For this review, take the finished solid that the model builds, in its own axes (mm). A direction names the side the tool comes from. Round coordinates to 2 decimals unless told otherwise and drop trailing zeros. Loops run counter-clockwise (first coordinate to the right, second up) from the corner with the lowest first, then second, coordinate; pieces in that order, holes last. Notation, with made-up numbers: M 70,-13.75 L 123,-13.75 A26 cw 123,6.25 Z; hole C 47,73 d8. An arc over 180 degrees is marked long. Write item = value, one per line. Start each with the question number.
Autodesk Inventor part; units mm, degrees
ref_plane "YZ Plane" through (0, 0, 0) normal (1, 0, 0) x (0, 1, 0)
ref_plane "XZ Plane" through (0, 0, 0) normal (0, 1, 0) x (-1, 0, 0)
ref_plane "XY Plane" through (0, 0, 0) normal (0, 0, 1) x (1, 0, 0)
sketch "Эскиз1" plane through (0, 0, 0) normal (0, 0, 1) x (1, 0, 0)
  line L0 (80, 0) -> (-80, 0) construction
  line L1 (80, 15) -> (-80, 15)
  line L2 (-80, -15) -> (80, -15)
  arc A0 (80, -15) -> (80, 15) centre (80, 0) ccw
  arc A1 (-80, 15) -> (-80, -15) centre (-80, 0) ccw
  circle A2 centre (0, 0) radius 12.5
  circle A3 centre (0, 0) radius 6
  circle A4 centre (-80, 0) radius 5
  circle A5 centre (80, 0) radius 5
  dimension "d0" = 80
  dimension "d1" = 30
  dimension "d4" = 25
  dimension "d5" = 12
  dimension "d6" = 10
  dimension "d7" = 10
extrude "Выдавливание1" add sketch "Эскиз1" against normal blind 10 contours A0 L2 A1 L1 | A2 | A3 | A4 | A5
extrude "Выдавливание2" cut sketch "Эскиз1" against normal blind 10 contours A5
extrude "Выдавливание3" cut sketch "Эскиз1" against normal blind 10 contours A4
extrude "Выдавливание4" add sketch "Эскиз1" along normal blind 20 contours A2
extrude "Выдавливание5" cut sketch "Эскиз1" along normal mid plane 2850 contours A3
equation "\"Глубина_просечки\" = 0.5 * Толщина"
properties part number "крышка" material "Сталь"
(1) Add section C-C on x = 0. Write out the cut boundary in (y, z).
(2) Add section B-B on y = 0. Write out the cut boundary in (x, z), and give its area (3 significant figures).
(3) Add section A-A on z = -3.25. Write out the cut boundary in (x, y).
(4) Wall thickness on L1, parallel to Y at x = -80, z = -6.5; L2, parallel to Z at x = -38.5, y = 8.75; L3, parallel to X at y = -2, z = 9.25: over which ranges is each line inside the solid? List them lowest first.
(5) For pin 1 Ø3 at (y, z) = (11, 3.5) entering from -X; pin 2 Ø10 at (x, y) = (53.5, -5.5) entering from +Z; pin 3 Ø1 at (y, z) = (-7, -2.5) entering from +X, all flat-tipped, find the tip position at first contact; note any pin that passes through.
(6) Add section D-D on z = 4.75. Write out the cut boundary in (x, y), and give its area (3 significant figures).
(7) Tool access review of faces 5 (the cylindrical face through (11.923, -3.755, 9.86)), 6 (the flat face through (1, 15, -5)): name each direction out of +Z, -Z, +X, -X, +Y, -Y from which nothing blocks a thin tool from reaching the whole face with its end or side.
(8) Draft analysis for pull direction Y (two halves, no side actions). For faces 1 (the cylindrical face through (84.619, -1.915, -4.93)), 2 (the flat face through (-1, -15, -5)), 3 (the flat face through (-3, -5.4, 20)), 4 (the cylindrical face through (-95, 0, -5)), state which applies: +Y half, -Y half, draft (parallel to the pull), parting line (faces both ways), or undercut.
Answer sheet:
q1.outline = M -15,-10 L -6,-10 L -6,20 L -12.5,20 L -12.5,0 L -15,0 Z; M 6,-10 L 15,-10 L 15,0 L 12.5,0 L 12.5,20 L 6,20 Z
q2.outline = M -95,-10 L -85,-10 L -85,0 L -95,0 Z; M -75,-10 L -6,-10 L -6,20 L -12.5,20 L -12.5,0 L -75,0 Z; M 6,-10 L 75,-10 L 75,0 L 12.5,0 L 12.5,20 L 6,20 Z; M 85,-10 L 95,-10 L 95,0 L 85,0 Z
q2.area = 1,840 mm²
q3.outline = M -80,-15 L 80,-15 A15 ccw 80,15 L -80,15 A15 ccw Z; hole C -80,0 d10; hole C 0,0 d12; hole C 80,0 d10
q4.L1 = -15 to -5, 5 to 15
q4.L2 = -10 to 0
q4.L3 = -12.34 to -5.66, 5.66 to 12.34
q5.pin_1 = -8.12
q5.pin_2 = 0
q5.pin_3 = 93.52
q6.outline = C 0,0 d25; hole C 0,0 d12
q6.area = 378 mm²
q7.face_5 = +Z
q7.face_6 = +Z, -Z, +X, -X, +Y
q8.face_1 = undercut
q8.face_2 = -Y half
q8.face_3 = draft
q8.face_4 = parting line
